Design review of the part built by this model. Coordinates are the model's own, in mm. Face numbers are marked on the shaded views. Round coordinates to 2 decimals unless told otherwise and drop trailing zeros. Order: outer loops, then holes, each group sorted by start corner. A loop starts at its lowest first (then second) coordinate and runs counter-clockwise, first axis right, second up. Notation, with made-up numbers: (11.5, 68.5) - (17.5, 68.5) arc R30 cw to (17.5, 104.5) - close; hole circle Ø1 at (26.25, 47.25). An arc over 180 degrees is marked (long way). Use CSV: the item, a comma, the result in double quotes. Start each with the question number.
from build123d import *

# Parameters (mm, degrees)
SKETCH1_R           = 52.5
BOSS_EXTRUDE1_DEPTH = 20
SKETCH2_R           = 42.5
SKETCH2_R_2         = 40
CUT_EXTRUDE1_DEPTH  = 7
FILLET1_R           = 5
SKETCH3_W           = 40
SKETCH3_H           = 3
SKETCH3_W_2         = 60
CUT_EXTRUDE2_DEPTH  = 10
SKETCH4_R           = 2.5
CUT_EXTRUDE3_DEPTH  = 5
SKETCH5_R           = 1.5
CUT_EXTRUDE4_DEPTH  = 15
SKETCH8_R           = 1.5
CUT_EXTRUDE5_DEPTH  = 15
SKETCH7_R           = 1.5
CUT_EXTRUDE6_DEPTH  = 15
SKETCH6_R           = 1.5
CUT_EXTRUDE7_DEPTH  = 15
SKETCH9_W           = 3
SKETCH9_H           = 10
CUT_EXTRUDE8_DEPTH  = 10
SKETCH10_R          = 2.5
CUT_EXTRUDE9_DEPTH  = 20
SKETCH11_W          = 50
SKETCH11_H          = 10
SKETCH11_R          = 3.25
BOSS_EXTRUDE2_DEPTH = 3
FILLET2_R           = 2.5


with BuildPart() as part:
    # Sketch1 → Boss-Extrude1 (new body)
    with BuildSketch(Plane.XY):
        Circle(SKETCH1_R)
    extrude(amount=BOSS_EXTRUDE1_DEPTH)

    # Sketch2 → Cut-Extrude1 (cut)
    with BuildSketch(Plane(origin=(0, 0, 0), x_dir=(-1, 0, 0), z_dir=(0, 0, -1))):
        Circle(SKETCH2_R)
        Circle(SKETCH2_R_2, mode=Mode.SUBTRACT)
    extrude(amount=-CUT_EXTRUDE1_DEPTH, mode=Mode.SUBTRACT)

    # Fillet1
    fillet1_edges = [part.edges().sort_by_distance(p)[0] for p in [
        (-52.5, 0, 20),
    ]]
    fillet(fillet1_edges, radius=FILLET1_R)

    # Sketch3 → Cut-Extrude2 (cut)
    with BuildSketch(Plane(origin=(0, 0, 0), x_dir=(-1, 0, 0), z_dir=(0, 0, -1))):
        with Locations((0, -23.5)):
            Rectangle(SKETCH3_W, SKETCH3_H)
        with Locations((0, 4.5)):
            Rectangle(SKETCH3_W_2, SKETCH3_H)
    extrude(amount=-CUT_EXTRUDE2_DEPTH, mode=Mode.SUBTRACT)

    # Sketch4 → Cut-Extrude3 (cut)
    with BuildSketch(Plane.XY.offset(20)):
        with Locations((0, 46.25)):
            Circle(SKETCH4_R)
        with Locations((46.25, 0)):
            Circle(SKETCH4_R)
        with Locations((0, -46.25)):
            Circle(SKETCH4_R)
        with Locations((-46.25, 0)):
            Circle(SKETCH4_R)
    extrude(amount=-CUT_EXTRUDE3_DEPTH, mode=Mode.SUBTRACT)

    # Sketch5 → Cut-Extrude4 (cut)
    with BuildSketch(Plane.XY.offset(15)):
        with Locations((0, 46.25)):
            Circle(SKETCH5_R)
    extrude(amount=-CUT_EXTRUDE4_DEPTH, mode=Mode.SUBTRACT)

    # Sketch8 → Cut-Extrude5 (cut)
    with BuildSketch(Plane.XY.offset(15)):
        with Locations((-46.25, 0)):
            Circle(SKETCH8_R)
    extrude(amount=-CUT_EXTRUDE5_DEPTH, mode=Mode.SUBTRACT)

    # Sketch7 → Cut-Extrude6 (cut)
    with BuildSketch(Plane.XY.offset(15)):
        with Locations((0, -46.25)):
            Circle(SKETCH7_R)
    extrude(amount=-CUT_EXTRUDE6_DEPTH, mode=Mode.SUBTRACT)

    # Sketch6 → Cut-Extrude7 (cut)
    with BuildSketch(Plane.XY.offset(15)):
        with Locations((46.25, 0)):
            Circle(SKETCH6_R)
    extrude(amount=-CUT_EXTRUDE7_DEPTH, mode=Mode.SUBTRACT)

    # Sketch9 → Cut-Extrude8 (cut)
    with BuildSketch(Plane(origin=(0, 0, 0), x_dir=(-1, 0, 0), z_dir=(0, 0, -1))):
        with Locations((0, -30)):
            Rectangle(SKETCH9_W, SKETCH9_H)
    extrude(amount=-CUT_EXTRUDE8_DEPTH, mode=Mode.SUBTRACT)

    # Sketch10 → Cut-Extrude9 (cut)
    with BuildSketch(Plane(origin=(0, 0, 0), x_dir=(-1, 0, 0), z_dir=(0, 0, -1))):
        with Locations((-20, 16)):
            Circle(SKETCH10_R)
        with Locations((-10, 16)):
            Circle(SKETCH10_R)
        with Locations((0, 16)):
            Circle(SKETCH10_R)
        with Locations((10, 16)):
            Circle(SKETCH10_R)
        with Locations((20, 16)):
            Circle(SKETCH10_R)
    extrude(amount=-CUT_EXTRUDE9_DEPTH, mode=Mode.SUBTRACT)

    # Sketch11 → Boss-Extrude2 (add)
    with BuildSketch(Plane.XY.offset(20)):
        with Locations((0, 16)):
            Rectangle(SKETCH11_W, SKETCH11_H)
        with Locations((-20, 16)):
            Circle(SKETCH11_R, mode=Mode.SUBTRACT)
        with Locations((-10, 16)):
            Circle(SKETCH11_R, mode=Mode.SUBTRACT)
        with Locations((0, 16)):
            Circle(SKETCH11_R, mode=Mode.SUBTRACT)
        with Locations((10, 16)):
            Circle(SKETCH11_R, mode=Mode.SUBTRACT)
        with Locations((20, 16)):
            Circle(SKETCH11_R, mode=Mode.SUBTRACT)
    extrude(amount=BOSS_EXTRUDE2_DEPTH)

    # Fillet2
    fillet2_edges = [part.edges().sort_by_distance(p)[0] for p in [
        (25, 11, 21.5),
        (25, 21, 21.5),
        (-25, 21, 21.5),
        (-25, 11, 21.5),
    ]]
    fillet(fillet2_edges, radius=FILLET2_R)


solid = part.part
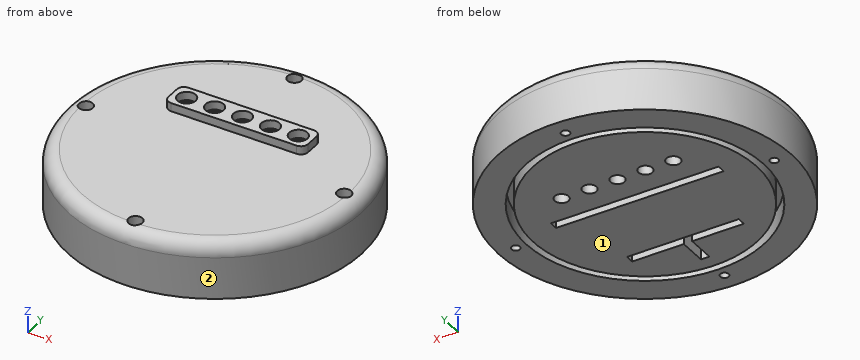
Q1. The part is to be moulded in two halves that separate along X. For the marked faces 1 and 2, say which applies: +X half, -X half, draft (parallel to the pull), parting line (faces both ways), or undercut.
Q2. For L1, parallel to X at y = 0, z = 18.7; L2, parallel to X at y = 7, z = 1.5; L3, parallel to Y at x = -7, z = 7.5, list the stretches that pass through material, from the lowest coordinate up. Write a range as [from, to].
Q3. Take a section at A-A (z = 2.25). Give the number of separate pieces and of enclosed holes in the cut face, plus the area to 3 significant figures.
Q4. Clearance check with flat-ended pins moving along their axes: pin 1 (8 mm diameter, centred on x = 0, y = -46.25, fed in from -Z); pin 2 (5 mm diameter, centred on x = 37.5, y = -32, fed in from +Z); pin 3 (0.9 mm diameter, centred on y = 15.5, z = 21, fed in from -X); pin 4 (1.5 mm diameter, centred on x = 0, y = 45, fed in from +Z). State where each tip first meets the part, or that it passes through.
Q5. Take a section at C-C (y = 0). State the section outline as (x, z) points.
Findings below:
1,face 1,"draft"
1,face 2,"parting line"
2,L1,"x = [-50.86, -48.75], [-43.75, 43.75], [48.75, 50.86]"
2,L2,"x = [-52.03, -41.92], [-39.38, 39.38], [41.92, 52.03]"
2,L3,"y = [-52.03, -25], [-22, 3], [6, 52.03]"
3,separate pieces,"2"
3,enclosed holes,"12"
3,area,"7,550 mm^2"
4,pin 1,"stops at z = 0"
4,pin 2,"stops at z = 20"
4,pin 3,"stops at x = -25"
4,pin 4,"stops at z = 15"
5,outline,"(-52.5, 0) - (-47.75, 0) - (-47.75, 15) - (-48.75, 15) - (-48.75, 19.84) arc R5 ccw to (-52.5, 15) - close; (-44.75, 0) - (-42.5, 0) - (-42.5, 7) - (-40, 7) - (-40, 0) - (40, 0) - (40, 7) - (42.5, 7) - (42.5, 0) - (44.75, 0) - (44.75, 15) - (43.75, 15) - (43.75, 20) - (-43.75, 20) - (-43.75, 15) - (-44.75, 15) - close; (47.75, 0) - (52.5, 0) - (52.5, 15) arc R5 ccw to (48.75, 19.84) - (48.75, 15) - (47.75, 15) - close"
